```python
from build123d import *

# Parameters (mm, degrees)
SKETCH1_W                      = 192.4
SKETCH1_H                      = 192.4
BOSS_EXTRUDE1_DEPTH            = 6.35
BOSS_EXTRUDE2_DEPTH            = 40
CBORE_FOR_M4_SHCS1_D           = 4.5
CBORE_FOR_M4_SHCS1_DEPTH       = 6.35
CBORE_FOR_M4_SHCS1_CBORE_D     = 8
CBORE_FOR_M4_SHCS1_CBORE_DEPTH = 4
CHAMFER1_SIZE                  = 1


with BuildPart() as part:
    # Sketch1 → Boss-Extrude1 (new body)
    with BuildSketch(Plane(origin=(0, 0, 0), x_dir=(1, 0, 0), z_dir=(0, 1, 0))):
        Rectangle(SKETCH1_W, SKETCH1_H)
    extrude(amount=BOSS_EXTRUDE1_DEPTH)

    # Sketch2 → Boss-Extrude2 (add)
    with BuildSketch(Plane(origin=(0, 6.35, 0), x_dir=(1, 0, 0), z_dir=(0, 1, 0))):
        Polygon((-92.2, 92.2), (-92.2, -92.2), (92.2, -92.2), (96.2, -92.2), (96.2, -96.2), (-96.2, -96.2), (-96.2, 96.2), (-92.2, 96.2), align=None)
    extrude(amount=BOSS_EXTRUDE2_DEPTH)

    # CBORE for M4 SHCS1
    with Locations(Plane(origin=(0, 6.35, 0), x_dir=(1, 0, 0), z_dir=(0, 1, 0))):
        with Locations((96.2, -76.2), (-76.2, -76.2), (-76.2, 75.92365398)):
            CounterBoreHole(CBORE_FOR_M4_SHCS1_D / 2, CBORE_FOR_M4_SHCS1_CBORE_D / 2, CBORE_FOR_M4_SHCS1_CBORE_DEPTH, depth=CBORE_FOR_M4_SHCS1_DEPTH)

    # Chamfer1
    chamfer1_edges = [part.edges().sort_by_distance(p)[0] for p in [
        (96.2, 0, -11.125),
        (0, 0, -96.2),
        (96.2, 0, 87.325),
    ]]
    chamfer(chamfer1_edges, length=CHAMFER1_SIZE)


solid = part.part
```
Can you work these out from the model? Positions are in its coordinate system, mm. A direction names the side the tool comes from. Round coordinates to 2 decimals unless told otherwise and drop trailing zeros. Loops run counter-clockwise (first coordinate to the right, second up) from the corner with the lowest first, then second, coordinate; pieces in that order, holes last.
Item 1: Suppose I cut it at D-D, the plane y = 31.5. Write out the boundary of the cut face in (x, z).
Item 2: Suppose I cut it at B-B, the plane z = -67. Write out the boundary of the cut face in (x, y), then the cut area to 3 significant figures.
Item 3: Please list where these lines run through material, in increasing order: L1, parallel to Z at x = -76.2, y = 3.6; L2, parallel to X at y = 1, z = 76; L3, parallel to X at y = 5.25, z = 76.2.
Item 4: If we mould it in two halves opening along Z, with no side actions, what happens to faces 4 (the flat face through (-74, 2.35, 78)), 5 (the flat face through (-96.2, 23, 1)), 6 (the flat face through (3, 26, 92.2)), 7 (the flat face through (1, 23, 96.2))? For each: +Z half, -Z half, draft (parallel to the pull), parting line (faces both ways), or undercut.
Item 5: Suppose I cut it at C-C, the plane x = 47. Write out the boundary of the cut face in (y, z), then the cut area to 3 significant figures.
Item 6: Will these pins go through, and if not, where does the flat tip stop? pin 1 Ø9 at (x, z) = (-76.2, 76.2) entering from +Y; pin 2 Ø4 at (y, z) = (37.5, 13.5) entering from +X; pin 3 Ø2 at (x, z) = (93.5, 77) entering from +Y; pin 4 Ø2.5 at (x, z) = (-76.2, 76.2) entering from -Y.
Item 7: Suppose I cut it at A-A, the plane x = -76.2. Write out the boundary of the cut face in (y, z).
Item 8: Which directions (+Z, -Z, +X, -X, +Y, -Y) give clear straight access to the entire face, cutting with the end or side of a thin tool? Please do faces 1 (the flat face through (1, 6.35, -3)), 2 (the cylindrical face through (-73.952, 1.159, -76.023)), 3 (the cylindrical face through (-79.4, 4.4, 78.6)).
Reported:
1. outline: (-96.2, -96.2) - (-92.2, -96.2) - (-92.2, 92.2) - (96.2, 92.2) - (96.2, 96.2) - (-96.2, 96.2) - close
2. outline: (-96.2, 0) - (95.2, 0) - (96.2, 1) - (96.2, 6.35) - (-92.2, 6.35) - (-92.2, 46.35) - (-96.2, 46.35) - close
2. area: 1,380 mm2
3. L1: z = -96.2 to -79.92, -71.92 to 72.2, 80.2 to 96.2
3. L2: x = -96.2 to -78.44, -73.96 to 93.96
3. L3: x = -96.2 to -80.2, -72.2 to 92.2
4. face 4: undercut
4. face 5: draft
4. face 6: -Z half
4. face 7: +Z half
5. outline: (0, -95.2) - (1, -96.2) - (6.35, -96.2) - (6.35, 92.2) - (46.35, 92.2) - (46.35, 96.2) - (0, 96.2) - close
5. area: 1,380 mm2
6. pin 1: stops at y = 6.35
6. pin 2: stops at x = -92.2
6. pin 3: stops at y = 2.35
6. pin 4: passes through
7. outline: (0, -95.2) - (1, -96.2) - (6.35, -96.2) - (6.35, -79.92) - (2.35, -79.92) - (2.35, -78.17) - (0, -78.17) - close; (0, -73.67) - (2.35, -73.67) - (2.35, -71.92) - (6.35, -71.92) - (6.35, 72.2) - (2.35, 72.2) - (2.35, 73.95) - (0, 73.95) - close; (0, 78.45) - (2.35, 78.45) - (2.35, 80.2) - (6.35, 80.2) - (6.35, 92.2) - (46.35, 92.2) - (46.35, 96.2) - (0, 96.2) - close
8. face 1: -Z, +X, +Y
8. face 2: +Y, -Y
8. face 3: +Y
